```python
from build123d import *

# Parameters (mm, degrees)
BOSS_EXTRUDE1_DEPTH = 200
CUT_EXTRUDE1_DEPTH  = 4
CHAMFER1_SIZE       = 3
SKETCH3_R           = 1.6
CUT_EXTRUDE2_DEPTH  = 3
CHAMFER2_SIZE       = 0.75


with BuildPart() as part:
    # Sketch1 → Boss-Extrude1 (new body)
    with BuildSketch(Plane.XY):
        Polygon((0, 0), (0, 48), (29, 48), (29, 23), (25, 23), (25, 44), (4, 44), (4, 0), (10.5, 0), (10.5, -3), (-6.5, -3), (-6.5, 0), align=None)
    extrude(amount=-BOSS_EXTRUDE1_DEPTH)

    # Sketch2 → Cut-Extrude1 (cut)
    with BuildSketch(Plane(origin=(29, 0, 0), x_dir=(0, 0, -1), z_dir=(1, 0, 0))):
        with BuildLine():
            Line((15, 36), (84.75, 36))
            ThreePointArc((84.75, 36), (86.164213562, 35.414213562), (86.75, 34))
            Line((86.75, 34), (86.75, 33))
            ThreePointArc((86.75, 33), (86.164213562, 31.585786438), (84.75, 31))
            Line((84.75, 31), (15, 31))
            ThreePointArc((15, 31), (13.585786438, 31.585786438), (13, 33))
            Line((13, 33), (13, 34))
            ThreePointArc((13, 34), (13.585786438, 35.414213562), (15, 36))
        make_face()
        with BuildLine():
            Line((114.75, 36), (185, 36))
            ThreePointArc((185, 36), (186.414213562, 35.414213562), (187, 34))
            Line((187, 34), (187, 33))
            ThreePointArc((187, 33), (186.414213562, 31.585786438), (185, 31))
            Line((185, 31), (114.75, 31))
            ThreePointArc((114.75, 31), (113.335786438, 31.585786438), (112.75, 33))
            Line((112.75, 33), (112.75, 34))
            ThreePointArc((112.75, 34), (113.335786438, 35.414213562), (114.75, 36))
        make_face()
    extrude(amount=-CUT_EXTRUDE1_DEPTH, mode=Mode.SUBTRACT)

    # Chamfer1
    chamfer1_edges = [part.edges().sort_by_distance(p)[0] for p in [
        (29, 31.585786438, -186.414213562),
        (29, 33.5, -187),
        (29, 35.414213562, -186.414213562),
        (29, 36, -149.875),
        (29, 35.414213562, -113.335786438),
        (29, 33.5, -112.75),
        (29, 31.585786438, -113.335786438),
        (29, 31, -149.875),
        (29, 31.585786438, -86.164213562),
        (29, 33.5, -86.75),
        (29, 35.414213562, -86.164213562),
        (29, 36, -49.875),
        (29, 35.414213562, -13.585786438),
        (29, 33.5, -13),
        (29, 31.585786438, -13.585786438),
        (29, 31, -49.875),
    ]]
    chamfer(chamfer1_edges, length=CHAMFER1_SIZE)

    # Sketch3 → Cut-Extrude2 (cut)
    with BuildSketch(Plane.XZ.offset(3)):
        with Locations((-3.25, -40)):
            Circle(SKETCH3_R)
        with Locations(Location((-3.25, -160, 0), (0, 0, 180))):
            Circle(SKETCH3_R)
        with Locations((7.25, -160)):
            Circle(SKETCH3_R)
        with Locations(Location((7.25, -40, 0), (0, 0, 180))):
            Circle(SKETCH3_R)
    extrude(amount=-CUT_EXTRUDE2_DEPTH, mode=Mode.SUBTRACT)

    # Chamfer2
    chamfer2_edges = [part.edges().sort_by_distance(p)[0] for p in [
        (8.85, 0, -40),
        (5.65, 0, -160),
        (-1.65, 0, -160),
        (-4.85, 0, -40),
    ]]
    chamfer(chamfer2_edges, length=CHAMFER2_SIZE)


solid = part.part
```
Part model, mm, in its own coordinate system. A direction names the side the tool comes from. Round coordinates to 2 decimals unless told otherwise and drop trailing zeros. Order: outer loops, then holes, each group sorted by start corner. A loop starts at its lowest first (then second) coordinate and runs counter-clockwise, first axis right, second up. Notation, with made-up numbers: M 1.5,47 L 54.5,47 A14 cw 54.5,57 Z; hole C -32,-4 d7. An arc over 180 degrees is marked long. Put each result on its own line as item: value. Start each with the question number.
1. Tool access for faces 4 (the face through (4, 22, -99)), 5 (the face through (27.146, 36.2, -112.501)), 6 (the face through (6.51, -1.89, -38.58)), 7 (the face through (-3, 0, -99)), 8 (the face through (14, 48, -99)): list every direction of +Z, -Z, +X, -X, +Y, -Y with a clear straight run to the whole face (end or side of a thin tool).
2. Slice it at C-C on y = 13. List the corners of the cut face in (x, z), then the cut area to 3 significant figures.
3. Slice it at A-A on z = -52. List the corners of the cut face in (x, y), then the cut area to 3 significant figures.
4. Slice it at B-B on z = -92. List the corners of the cut face in (x, y), then the cut area to 3 significant figures.
5. Drill centre lines: probe 1 along Z at (x, y) = (-3.25, -2.2); probe 2 along X at (y, z) = (-1.9, -160); probe 3 along X at (y, z) = (28, -52). Where is each one in solid material? Low to high. Write a range as [from, to].
6. Two-plate mould, pull along X, no slides. Class faces 1 (the face through (3, 26, -200)), 2 (the face through (27.146, 36.249, -86.95)), 3 (the face through (25, 33, -99)): +X half, -X half, draft (parallel to the pull), parting line (faces both ways), or undercut.
7. Drop flat-ended pins along their axis: pin 1 (1 mm diameter, centred on y = 6, z = -89, fed in from +X); pin 2 (1 mm diameter, centred on y = 26, z = -178.5, fed in from -X); pin 3 (3.5 mm diameter, centred on y = -2, z = -144, fed in from +X). Give the stop position or say it passes through.
Findings:
1. face 4: +Z, -Z
1. face 5: +X
1. face 6: -Y
1. face 7: +Z, -Z, -X, +Y
1. face 8: +Z, -Z, +X, -X, +Y
2. outline: M 0,-200 L 4,-200 L 4,0 L 0,0 Z
2. area: 800 mm2
3. outline: M -6.5,-3 L 10.5,-3 L 10.5,0 L 4,0 L 4,44 L 25,44 L 25,36 L 26,36 L 29,39 L 29,48 L 0,48 L 0,0 L -6.5,0 Z; M 25,23 L 29,23 L 29,28 L 26,31 L 25,31 Z
3. area: 398 mm2
4. outline: M -6.5,-3 L 10.5,-3 L 10.5,0 L 4,0 L 4,44 L 25,44 L 25,23 L 29,23 L 29,48 L 0,48 L 0,0 L -6.5,0 Z
4. area: 427 mm2
5. probe 1: [-200, -161.6], [-158.4, -41.6], [-38.4, 0]
5. probe 2: [-6.5, -4.85], [-1.65, 5.65], [8.85, 10.5]
5. probe 3: [0, 4], [25, 29]
6. face 1: draft
6. face 2: +X half
6. face 3: undercut
7. pin 1: x = 4
7. pin 2: x = 0
7. pin 3: x = 10.5
